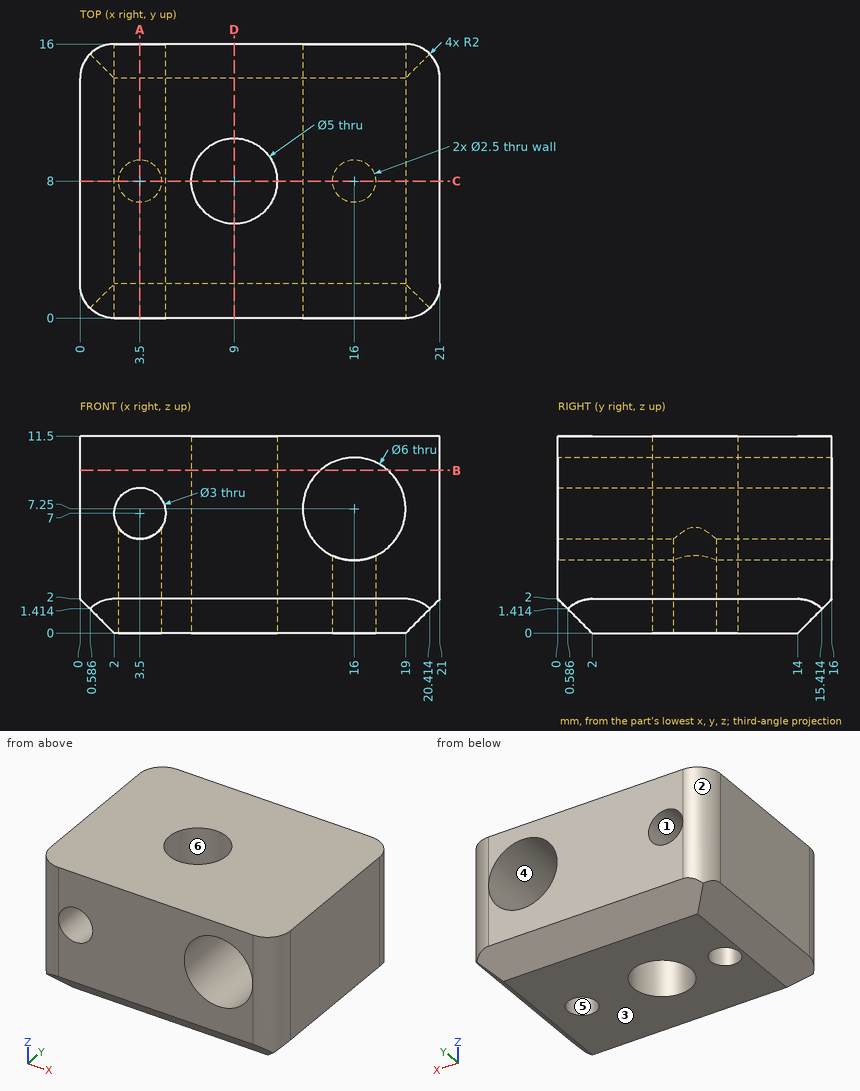
Could you check a few things on this drawing? It's one solid part, dimensions in mm from its lowest x, y, z. A direction names the side the tool comes from. Coordinates: 2 decimals unless noted, no trailing zeros. Write each loop counter-clockwise with the first axis right and the second up, starting at its lowest first coordinate (ties: lowest second). Pieces come first, ordered by that corner, then holes. Notation, with made-up numbers: (8.5, 1.5) - (48.5, 1.5) arc R19 ccw to (48.5, 31.5) - close; hole circle Ø3 at (-33, -34). An arc over 180 degrees is marked (long way). Return JSON: item names as keys, results as strings. Group by question number.
Item 1: If we section it at C-C (y = 8): Write out the boundary of the cut face in (x, z).
Item 2: Please list where these lines run through material, in increasing order: probe 1 along X at (y, z) = (2.25, 6); probe 2 along Y at (x, z) = (3.5, 2.25); probe 3 along Z at (x, y) = (18, 10) (1 decimal).
Item 3: If we section it at D-D (x = 9): Write out the boundary of the cut face in (y, z), then the cut area to 4 significant figures.
Item 4: Which directions (+Z, -Z, +X, -X, +Y, -Y) give clear straight access to the entire face, cutting with the end or side of a thin tool? Please do the marked faces 5 and 6.
Item 5: If we section it at B-B (z = 9.5): Write out the boundary of the cut face in (x, y).
Item 6: We'd pull the mould along Z, two halves only. Please class the marked faces 1, 2, 3 and 4: pulls with the +Z half, pulls with the -Z half, needs draft (parallel to the pull), parting line crosses it, or undercut.
Item 7: If we section it at A-A (x = 3.5): Write out the boundary of the cut face in (y, z).
Return value:
{
 "1": {"outline": "(0, 2) - (2, 0) - (2.25, 0) - (2.25, 6.17) arc R1.5 cw (long way) to (4.75, 6.17) - (4.75, 0) - (6.5, 0) - (6.5, 11.5) - (0, 11.5) - close; (11.5, 0) - (14.75, 0) - (14.75, 4.52) arc R3 cw (long way) to (17.25, 4.52) - (17.25, 0) - (19, 0) - (21, 2) - (21, 11.5) - (11.5, 11.5) - close"},
 "2": {"probe 1": "x = 0 to 2.38, 4.62 to 13.27, 18.73 to 21", "probe 2": "y = 0 to 6.75, 9.25 to 16", "probe 3": "z = 0 to 5, 9.5 to 11.5"},
 "3": {"outline": "(0, 2) - (2, 0) - (5.5, 0) - (5.5, 11.5) - (0, 11.5) - close; (10.5, 0) - (14, 0) - (16, 2) - (16, 11.5) - (10.5, 11.5) - close", "area": "122.5 mm^2"},
 "4": {"face 5": "-Z", "face 6": "+Z, -Z"},
 "5": {"outline": "(0, 2) arc R2 ccw to (2, 0) - (14.02, 0) - (14.02, 16) - (2, 16) arc R2 ccw to (0, 14) - close; (17.98, 0) - (19, 0) arc R2 ccw to (21, 2) - (21, 14) arc R2 ccw to (19, 16) - (17.98, 16) - close; hole circle Ø5 at (9, 8)"},
 "6": {"face 1": "undercut", "face 2": "needs draft", "face 3": "pulls with the -Z half", "face 4": "undercut"},
 "7": {"outline": "(0, 2) - (2, 0) - (6.75, 0) - (6.75, 5.5) - (0, 5.5) - close; (0, 8.5) - (16, 8.5) - (16, 11.5) - (0, 11.5) - close; (9.25, 0) - (14, 0) - (16, 2) - (16, 5.5) - (9.25, 5.5) - close"}
}
